Check sheet for the modelled part. Datum: model origin and axes. Units: mm. Coordinates: 2 decimals unless noted, no trailing zeros. Loops run counter-clockwise (first coordinate to the right, second up) from the corner with the lowest first, then second, coordinate; pieces in that order, holes last. Notation, with made-up numbers: (16, 51) - (37, 51) arc R25 ccw to (37, 87) - close; hole circle Ø11 at (31, -20.75). An arc over 180 degrees is marked (long way). Write each question's results on one line, items separated by ' | '. Start each with the question number.
1. Cross-section at A-A (y = 18.5). Record the cut outline in (x, z) (3 decimals), and give its area (4 significant figures).
2. Gauge pin test, flat end, axial feed: P1, Ø3.5, axis at x = 46, y = 23, coming from the +Z side. Record the tip position at first contact, or that the pin passes through.
3. Draft check along X on faces 1 (the face through (35.908, -22.399, 1.61)), 2 (the face through (1, 27, 2)), 3 (the face through (-54, 0, 2)). Enter one of: released by +X, released by -X, zero draft, split by the parting line, or undercut.
4. Cross-section at D-D (z = 1.7). Give the number of separate pieces and of enclosed holes in the cut face, and give its area (3 significant figures).
5. Thickness scan on line 1 (Y direction, x = -34, z = 1.3); line 2 (X direction, y = -15, z = 1.5); line 3 (X direction, y = 9.5, z = 1.65). Record the ranges inside material, lowest first. Write a range as [from, to].
6. Cross-section at C-C (y = -23). Record the cut outline in (x, z) (3 decimals), and give its area (3 significant figures).
7. Cross-section at B-B (x = -34). Record the cut outline in (y, z) (3 decimals).
Autodesk Inventor part; units mm, degrees
ref_plane "YZ Plane" through (0, 0, 0) normal (1, 0, 0) x (0, 1, 0)
ref_plane "XZ Plane" through (0, 0, 0) normal (0, 1, 0) x (-1, 0, 0)
ref_plane "XY Plane" through (0, 0, 0) normal (0, 0, 1) x (1, 0, 0)
sketch "Sketch1" plane through (0, 0, 0) normal (0, 0, 1) x (1, 0, 0)
  line L0 (-54, -27) -> (54, -27)
  line L1 (54, -27) -> (54, 27)
  line L2 (54, 27) -> (-54, 27)
  line L3 (-54, 27) -> (-54, -27)
  line L4 (-54, -27) -> (54, 27) construction
  line L5 (54, -27) -> (-54, 27) construction
  point P0 (0, 0)
  dimension "d0" = 108
  dimension "d1" = 54
extrude "Extrusion1" add sketch "Sketch1" along normal blind 3.175
sketch "Sketch2" plane through (0, 0, 3.175) normal (0, 0, 1) x (1, 0, 0)
  line L0 (-54, -27) -> (54, -27) construction
  line L1 (54, -27) -> (54, 27) construction
  line L2 (54, 27) -> (-54, 27) construction
  line L3 (-54, 27) -> (-54, -27) construction
  line L4 (-54, -27) -> (54, -27)
  line L5 (0, 27) -> (0, -27) construction
  circle A0 centre (-40, -17) radius 2.5
  circle A1 centre (-46, -23) radius 2
  circle A2 centre (-34, -23) radius 2
  circle A3 centre (-34, -11) radius 2
  circle A4 centre (-46, -11) radius 2
  circle A5 centre (40, -17) radius 2.5
  circle A6 centre (46, -23) radius 2
  circle A7 centre (34, -23) radius 2
  circle A8 centre (34, -11) radius 2
  circle A9 centre (46, -11) radius 2
  line L6 (-54, 0) -> (54, 0) construction
  circle A10 centre (-40, 17) radius 2.5
  circle A11 centre (-46, 23) radius 2
  circle A12 centre (-34, 23) radius 2
  circle A13 centre (-34, 11) radius 2
  circle A14 centre (-46, 11) radius 2
  circle A15 centre (34, 11) radius 2
  circle A16 centre (34, 23) radius 2
  circle A17 centre (40, 17) radius 2.5
  circle A18 centre (46, 11) radius 2
  circle A19 centre (46, 23) radius 2
  point P0 (0, 0)
  point P1 (0, 0)
  point P2 (0, 0)
  dimension "d11" = 5
  dimension "d12" = 40
  dimension "d13" = 10
  dimension "d14" = 4
  dimension "d15" = 6
  dimension "d16" = 6
  dimension "d19" = 360
extrude "Extrusion2" cut sketch "Sketch2" against normal through all
properties part number "TurretMotorPlate"
Established:
1) outline: (-54, 0) - (-42, 0) - (-42, 3.175) - (-54, 3.175) - close; (-38, 0) - (38, 0) - (38, 3.175) - (-38, 3.175) - close; (42, 0) - (54, 0) - (54, 3.175) - (42, 3.175) - close | area: 317.5 mm^2
2) P1: through
3) face 1: undercut | face 2: zero draft | face 3: released by -X
4) separate pieces: 1 | enclosed holes: 20 | area: 5,550 mm^2
5) line 1: [-27, -25], [-21, -13], [-9, 9], [13, 21], [25, 27] | line 2: [-54, -41.5], [-38.5, 38.5], [41.5, 54] | line 3: [-54, -47.32], [-44.68, -35.32], [-32.68, 32.68], [35.32, 44.68], [47.32, 54]
6) outline: (-54, 0) - (-48, 0) - (-48, 3.175) - (-54, 3.175) - close; (-44, 0) - (-36, 0) - (-36, 3.175) - (-44, 3.175) - close; (-32, 0) - (32, 0) - (32, 3.175) - (-32, 3.175) - close; (36, 0) - (44, 0) - (44, 3.175) - (36, 3.175) - close; (48, 0) - (54, 0) - (54, 3.175) - (48, 3.175) - close | area: 292 mm^2
7) outline: (-27, 0) - (-25, 0) - (-25, 3.175) - (-27, 3.175) - close; (-21, 0) - (-13, 0) - (-13, 3.175) - (-21, 3.175) - close; (-9, 0) - (9, 0) - (9, 3.175) - (-9, 3.175) - close; (13, 0) - (21, 0) - (21, 3.175) - (13, 3.175) - close; (25, 0) - (27, 0) - (27, 3.175) - (25, 3.175) - close
